Build history of the part. All positions in model axes, mm. A direction names the side the tool comes from. Give positions to 0.01 mm unless a question says otherwise; leave off trailing zeros. Order: outer loops, then holes, each group sorted by start corner. A loop starts at its lowest first (then second) coordinate and runs counter-clockwise, first axis right, second up. Notation, with made-up numbers: M 75.25,10.5 L 94.25,10.5 A19 ccw 94.25,41.5 Z; hole C 3,40 d5. An arc over 180 degrees is marked long. Use CSV: the item, a comma, the result in double quotes. Start each with the question number.
Item 1: Band-saw the part on A-A on z = -47. Write the cut outline in (x, y).
Item 2: Pin check, flat tips, straight feed: P1, Ø2, axis at y = 2.5, z = -46.5, coming from the +X side; P2, Ø2, axis at x = 94.5, y = 2, coming from the -Z side; P3, Ø1.2, axis at y = 2, z = 1, coming from the -X side. Stop position of each tip, or through.
Item 3: Two-plate mould, pull along X, no slides. Class faces 1 (the flat face through (74, 2, 0)), 2 (the flat face through (58, 2, -30)), 3 (the flat face through (0, 2, -9)), 4 (the flat face through (39, 2, -40)): pulls with the +X half, pulls with the -X half, needs draft (parallel to the pull), parting line crosses it, or undercut.
Item 4: Band-saw the part on C-C on z = -19. Write the cut outline in (x, y), plus the area to 3 significant figures.
Item 5: Band-saw the part on B-B on x = 52. Write the cut outline in (y, z).
Item 6: Wall check: line 1 along Z through (x, y) = (51, 2.2); line 2 along Z through (x, y) = (43.5, 2.45); line 3 along Z through (x, y) = (35, 3.4). Give the ranges that are in metal, low to high.
Item 7: Which spindle directions (+Z, -Z, +X, -X, +Y, -Y) get a long thin tool onto all of the face, cutting with end or side? Do faces 5 (the flat face through (48, 2, -34)), 6 (the flat face through (53, 2, -44)), 7 (the flat face through (96, 2, -28)). Say none if no direction does.
Item 8: Band-saw the part on D-D on x = 73. Write the cut outline in (y, z).
from build123d import *

# Parameters (mm, degrees)
SKETCH_1_W      = 4
SKETCH_1_H      = 20
SKETCH_1_W_2    = 20
SKETCH_1_H_2    = 4
EXTRUDE_2_DEPTH = 4


with BuildPart() as part:
    # 草图1 → 凸台-拉伸2 (new body)
    with BuildSketch(Plane(origin=(0, 0, 0), x_dir=(1, 0, 0), z_dir=(0, 1, 0))):
        Polygon((0, 18), (0, 0), (36, 0), (56, 0), (92, 0), (92, 18), (92, 38), (92, 56), (48, 56), (48, 48), (58, 48), (58, 44), (48, 44), (48, 40), (58, 40), (58, 36), (48, 36), (48, 34), (48, 32), (58, 32), (58, 28), (48, 28), (48, 24), (58, 24), (58, 20), (48, 20), (48, 16), (58, 16), (58, 12), (48, 12), (44, 12), (44, 16), (34, 16), (34, 20), (44, 20), (44, 24), (34, 24), (34, 28), (44, 28), (44, 32), (34, 32), (34, 36), (44, 36), (44, 40), (34, 40), (34, 44), (44, 44), (44, 56), (0, 56), (0, 38), align=None)
        with Locations((-2, 28)):
            Rectangle(SKETCH_1_W, SKETCH_1_H)
        with Locations((46, -2)):
            Rectangle(SKETCH_1_W_2, SKETCH_1_H_2)
        with Locations((94, 28)):
            Rectangle(SKETCH_1_W, SKETCH_1_H)
    extrude(amount=EXTRUDE_2_DEPTH)


solid = part.part
Model answer:
1,outline,"M 0,0 L 44,0 L 44,4 L 0,4 Z; M 58,0 L 92,0 L 92,4 L 58,4 Z"
2,P1,"stops at x = 92"
2,P2,"stops at z = -38"
2,P3,"stops at x = 36"
3,face 1,"needs draft"
3,face 2,"undercut"
3,face 3,"pulls with the -X half"
3,face 4,"undercut"
4,outline,"M -4,0 L 34,0 L 34,4 L -4,4 Z; M 48,0 L 96,0 L 96,4 L 48,4 Z"
4,area,"344 mm^2"
5,outline,"M 0,-56 L 4,-56 L 4,-48 L 0,-48 Z; M 0,-44 L 4,-44 L 4,-40 L 0,-40 Z; M 0,-36 L 4,-36 L 4,-32 L 0,-32 Z; M 0,-28 L 4,-28 L 4,-24 L 0,-24 Z; M 0,-20 L 4,-20 L 4,-16 L 0,-16 Z; M 0,-12 L 4,-12 L 4,4 L 0,4 Z"
6,line 1,"z = -56 to -48, -44 to -40, -36 to -32, -28 to -24, -20 to -16, -12 to 4"
6,line 2,"z = -56 to -44, -40 to -36, -32 to -28, -24 to -20, -16 to 4"
6,line 3,"z = -56 to -44, -40 to -36, -32 to -28, -24 to -20, -16 to 0"
7,face 5,"-Z, +Y, -Y"
7,face 6,"+Y, -Y"
7,face 7,"+Z, -Z, +X, +Y, -Y"
8,outline,"M 0,-56 L 4,-56 L 4,0 L 0,0 Z"
